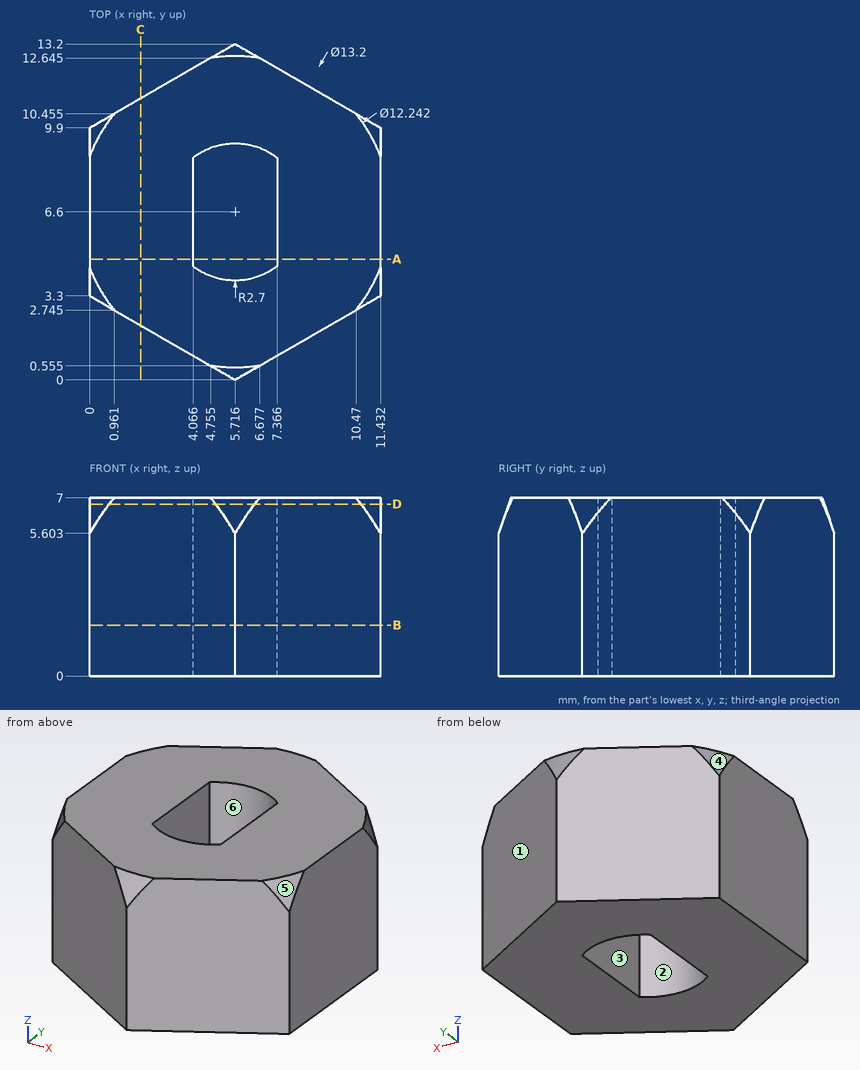
Design review of the part shown in the three views and the two pictorial views. Dimensions are in mm from the part's minimum x, y and z. A direction names the side the tool comes from. Give positions to 0.01 mm unless a question says otherwise; leave off trailing zeros. Loops run counter-clockwise (first coordinate to the right, second up) from the corner with the lowest first, then second, coordinate; pieces in that order, holes last. Notation, with made-up numbers: M 54.25,86.25 L 60.25,86.25 A32 ccw 60.25,124.25 Z; hole C 16,15 d10. An arc over 180 degrees is marked long. Put each result on its own line as item: value. Start each with the question number.
(1) The part is to be moulded in two halves that separate along X. For the marked faces 1, 2, 3 and 4, say which applies: +X half, -X half, draft (parallel to the pull), parting line (faces both ways), or undercut.
(2) Add section B-B, the plane z = 2. Write out the cut boundary in (x, y) (1 decimal).
(3) Machinability: for the marked faces 5 and 6, which of the approach directions +Z, -Z, +X, -X, +Y, -Y give a long, thin tool a straight path to every point of the face, cutting with its end or side? Answer none if there is none.
(4) Add section A-A, the plane y = 4.75. Write out the cut boundary in (x, z) (1 decimal).
(5) Wall thickness on L1, parallel to X at y = 8, z = 0.75 (1 decimal); L2, parallel to X at y = 12.25, z = 3.5 (1 decimal); L3, parallel to Y at x = 5, z = 5.25 (1 decimal): over which ranges is each line inside the solid? List them lowest first.
(6) Add section C-C, the plane x = 2. Write out the cut boundary in (y, z) (1 decimal).
(7) For pin 1 (1.5 mm diameter, centred on y = 11, z = 1, fed in from -X) (1 decimal), flat-tipped, find the tip position at first contact; note if it passes through.
(8) Add section D-D, the plane z = 6.75. Write out the cut boundary in (x, y) (1 decimal).
Result:
1. face 1: +X half
1. face 2: undercut
1. face 3: undercut
1. face 4: -X half
2. outline: M 0,3.3 L 5.7,0 L 11.4,3.3 L 11.4,9.9 L 5.7,13.2 L 0,9.9 Z; hole M 4.1,4.5 A2.7 ccw 7.4,4.5 L 7.4,8.7 A2.7 ccw 4.1,8.7 Z
3. face 5: +Z, +X, -Y
3. face 6: +Z, -Z
4. outline: M 0,0 L 4.1,0 L 4.1,7 L 0,7 Z; M 7.4,0 L 11.4,0 L 11.4,7 L 7.4,7 Z
5. L1: x = 0 to 4.1, 7.4 to 11.4
5. L2: x = 4.1 to 7.4
5. L3: y = 0.4 to 4, 9.2 to 12.8
6. outline: M 2.1,0 L 11.1,0 L 11.1,7 L 2.1,7 Z
7. pin 1: stops at x = 0.6
8. outline: M 0,4.2 A6.2 ccw 0.8,2.9 L 5,0.4 A6.2 ccw 6.5,0.4 L 10.7,2.9 A6.2 ccw 11.4,4.2 L 11.4,9 A6.2 ccw 10.7,10.3 L 6.5,12.8 A6.2 ccw 5,12.8 L 0.8,10.3 A6.2 ccw 0,9 Z; hole M 4.1,4.5 A2.7 ccw 7.4,4.5 L 7.4,8.7 A2.7 ccw 4.1,8.7 Z
